The listing builds one solid part. Answer for the finished solid, in the listing's coordinates (mm). Face numbers are marked on the shaded views. A direction names the side the tool comes from. Coordinates: 2 decimals unless noted, no trailing zeros. Order: outer loops, then holes, each group sorted by start corner. A loop starts at its lowest first (then second) coordinate and runs counter-clockwise, first axis right, second up.
Autodesk Inventor part; units mm, degrees
ref_plane "YZ Plane" through (0, 0, 0) normal (1, 0, 0) x (0, 1, 0)
ref_plane "XZ Plane" through (0, 0, 0) normal (0, 1, 0) x (-1, 0, 0)
ref_plane "XY Plane" through (0, 0, 0) normal (0, 0, 1) x (1, 0, 0)
sketch "Sketch1" plane through (0, 0, 0) normal (0, 0, 1) x (1, 0, 0)
  line L0 (3, 0) -> (33, 0)
  line L1 (33, 0) -> (33, 3)
  line L2 (33, 3) -> (3, 3)
  line L3 (3, 3) -> (3, 33)
  line L4 (3, 33) -> (0, 33)
  line L5 (0, 33) -> (0, 3)
  arc A0 (0, 3) -> (3, 0) centre (3, 3) ccw
  point P0 (0, 0)
extrude "Extrusion1" add sketch "Sketch1" along normal blind 26.5
sketch "Sketch2" plane through (3, 3, 0) normal (1, 0, 0) x (0, 0, -1)
  line L0 (0, 30) -> (-26.5, 30)
  circle A0 centre (-13.25, 16.75) radius 13.25
  line L1 (0, 0) -> (0, 30)
  circle A1 centre (-13.25, 16.75) radius 4
  line L2 (-21.75, 16.75) -> (-4.75, 16.75)
  circle A2 centre (-4.75, 16.75) radius 1.6
  circle A3 centre (-21.75, 16.75) radius 1.6
  line L3 (-26.5, 0) -> (-26.5, 30)
  point P0 (0, -3)
  point P1 (-26.5, 16.75)
  point P2 (-13.25, 30)
  point P3 (0, 16.75)
  dimension "d9" = 3.2
  dimension "d10" = 3.2
extrude "Extrusion2" cut sketch "Sketch2" against normal up to surface (3 mm away) contours L1 A0 L0 | A0 L3 L0 | L2 A1 | A3 | A1 L2 | A2
sketch "Sketch3" plane through (3, 3, 0) normal (0, 1, 0) x (1, 0, 0)
  line L0 (30, 0) -> (30, -26.5)
  line L1 (30, 0) -> (0, 0)
  line L2 (30, -26.5) -> (0, -26.5)
  line L3 (30, 0) -> (27, 0)
  arc A0 (30, -3) -> (27, 0) centre (27, -3) ccw
  arc A1 (27, -26.5) -> (30, -23.5) centre (27, -23.5) ccw
  circle A2 centre (15, -13.25) radius 5
  circle A3 centre (22, -5.25) radius 1.7
  circle A4 centre (8, -5.25) radius 1.7
  circle A5 centre (22, -21.25) radius 1.7
  circle A6 centre (8, -21.25) radius 1.7
  point P0 (-3, 0)
  point P1 (30, -23.5)
extrude "Extrusion3" cut sketch "Sketch3" against normal up to surface (3 mm away)
properties part number "do_ga"
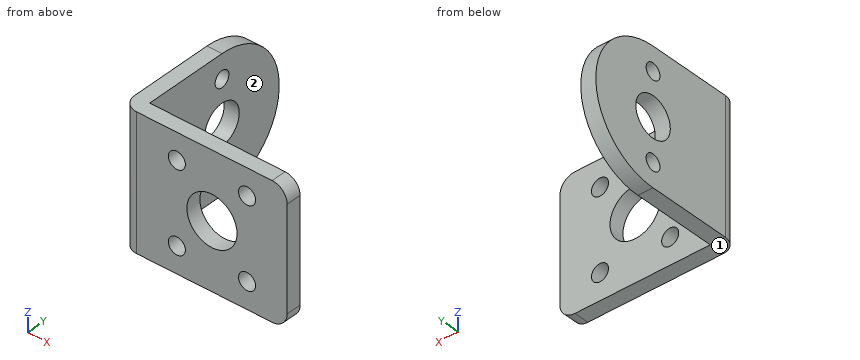
1) Each of these flat-tipped pins is pushed along its axis until it touches: P1, Ø8, axis at y = 12, z = 10, coming from the +X side; P2, Ø2, axis at x = 18.5, z = 6.5, coming from the +Y side. Where does it stop, or does it pass through?
2) A cutting plane is placed at D-D, the plane y = 23. Write down the section's boundary in (x, z), plus the area to 3 significant figures.
3) A cutting plane is placed at B-B, the plane z = 13.25. Write down the section's boundary in (x, y), plus the area to 3 significant figures.
4) A cutting plane is placed at C-C, the plane x = 25. Write down the section's boundary in (y, z).
5) Straight lines are drawn through the part: probe 1 along Z at (x, y) = (11, 1); probe 2 along X at (y, z) = (1.55, 21.25); probe 3 along Z at (x, y) = (18, 2.2). For each, find the intervals that lie inside material, in ascending order.
6) For the marked faces 1 and 2, determine the directions among +Z, -Z, +X, -X, +Y, -Y from which every point of the face is accessible in a straight line to the end or side of a thin tool.
7) A cutting plane is placed at A-A, the plane x = 18. Write down the section's boundary in (y, z), plus the area to 3 significant figures.
Working result:
1. P1: stops at x = 3
1. P2: stops at y = 3
2. outline: (0, 0.4) - (3, 0.4) - (3, 10.92) - (0, 10.92) - close; (0, 15.58) - (3, 15.58) - (3, 26.1) - (0, 26.1) - close
2. area: 63.1 mm2
3. outline: (0, 3) arc R3 ccw to (3, 0) - (13, 0) - (13, 3) - (3, 3) - (3, 15.75) - (0, 15.75) - close; (0, 23.75) - (3, 23.75) - (3, 33) - (0, 33) - close; (23, 0) - (33, 0) - (33, 3) - (23, 3) - close
3. area: 133 mm2
4. outline: (0, 0) - (3, 0) - (3, 3.55) - (0, 3.55) - close; (0, 6.95) - (3, 6.95) - (3, 19.55) - (0, 19.55) - close; (0, 22.95) - (3, 22.95) - (3, 26.5) - (0, 26.5) - close
5. probe 1: z = 0 to 3.55, 6.95 to 19.55, 22.95 to 26.5
5. probe 2: x = 0.37 to 9.3, 12.7 to 23.3, 26.7 to 33
5. probe 3: z = 0 to 8.25, 18.25 to 26.5
6. face 1: -Z, +X, -X, +Y, -Y
6. face 2: +Z, -Z, +X, +Y
7. outline: (0, 0) - (3, 0) - (3, 8.25) - (0, 8.25) - close; (0, 18.25) - (3, 18.25) - (3, 26.5) - (0, 26.5) - close
7. area: 49.5 mm2
